Drawing for the job (mm, zero at the part's lowest x, y, z). Give positions to 0.01 mm unless a question says otherwise; leave off trailing zeros. Order: outer loops, then holes, each group sorted by start corner. A loop starts at its lowest first (then second) coordinate and runs counter-clockwise, first axis right, second up. Notation, with made-up numbers: (74.25, -40) - (92.25, -40) arc R17 ccw to (92.25, -24) - close; hole circle Ø10 at (-31.75, -34.75). An arc over 180 degrees is marked (long way). One line per item, written item: value.
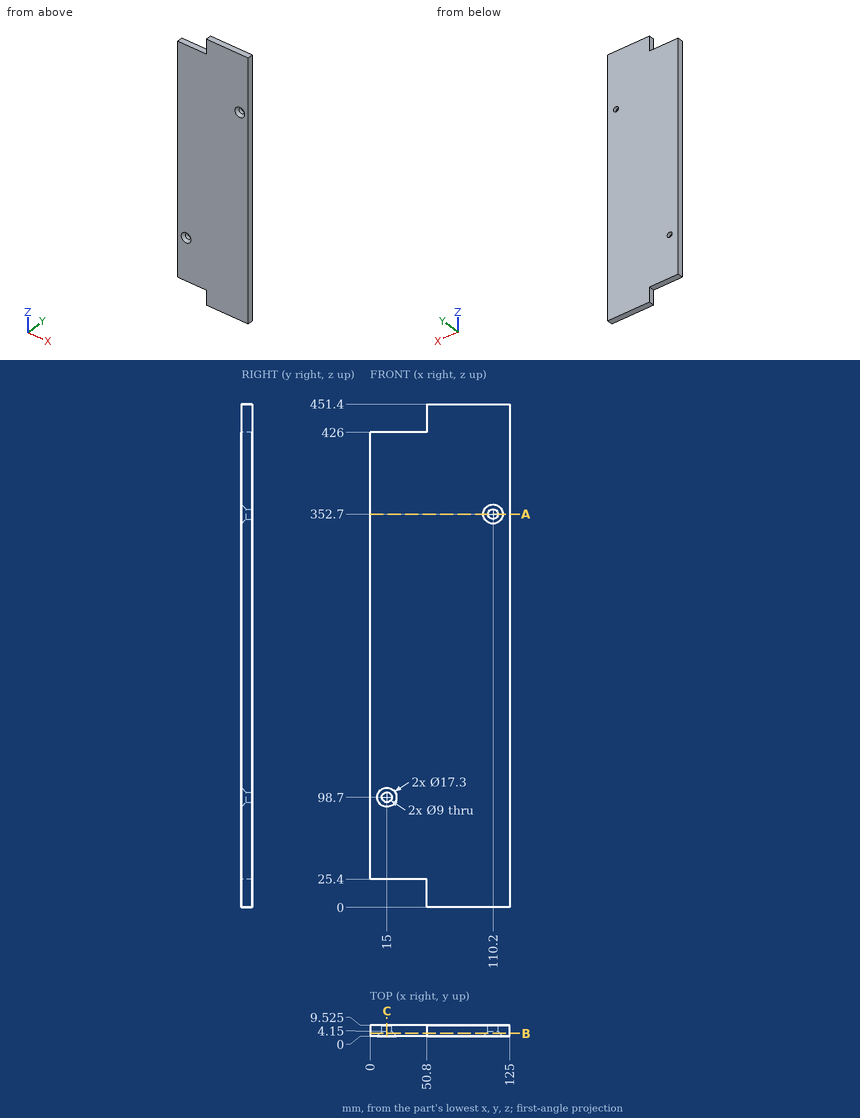
1) Cut at A-A, the plane z = 352.7. Give the cut face in (x, y) (3 decimals).
Outcome:
outline: (0, 0) - (101.55, 0) - (105.7, 4.15) - (105.7, 9.525) - (0, 9.525) - close; (114.7, 4.15) - (118.85, 0) - (125, 0) - (125, 9.525) - (114.7, 9.525) - close
2) Cut at C-C, the plane x = 15. Give the cut face in (y, z) (3 decimals), then the cut area to 3 significant figures.
Outcome:
outline: (0, 25.4) - (9.525, 25.4) - (9.525, 94.2) - (4.15, 94.2) - (0, 90.05) - close; (0, 107.35) - (4.15, 103.2) - (9.525, 103.2) - (9.525, 426) - (0, 426) - close
area: 3,710 mm^2
3) Pin check, flat tips, straight feed: pin 1 (5 mm diameter, centred on y = 5, z = 438, fed in from -X); pin 2 (10.5 mm diameter, centred on x = 110.2, z = 352.7, fed in from +Y) (3 decimals); pin 3 (5 mm diameter, centred on x = 31.5, y = 6.5, fed in from -Z); pin 4 (8 mm diameter, centred on x = 15, z = 98.7, fed in from +Y). Stop position of each tip, or through.
Outcome:
pin 1: stops at x = 50.8
pin 2: stops at y = 9.525
pin 3: stops at z = 25.4
pin 4: passes through
4) Drill centre lines: line 1 along X through (y, z) = (5.95, 98.7); line 2 along Z through (x, y) = (15, 6.9); line 3 along Z through (x, y) = (110.2, 7). Where is each one in solid material? Low to high. Write a range as from..to.
Outcome:
line 1: x = 0..10.5, 19.5..125
line 2: z = 25.4..94.2, 103.2..426
line 3: z = 0..348.2, 357.2..451.4
5) Cut at B-B, the plane y = 2.25. Give the cut face in (x, z).
Outcome:
outline: (0, 25.4) - (50.8, 25.4) - (50.8, 0) - (125, 0) - (125, 451.4) - (50.8, 451.4) - (50.8, 426) - (0, 426) - close; hole circle Ø12.8 at (15, 98.7); hole circle Ø12.8 at (110.2, 352.7)
